Read the model definition and answer for the solid it produces. Units are mm, in the model's axes. Face numbers are marked on the shaded views. A direction names the side the tool comes from. Coordinates: 2 decimals unless noted, no trailing zeros. Write each loop counter-clockwise with the first axis right and the second up, starting at its lowest first coordinate (ties: lowest second). Pieces come first, ordered by that corner, then holes.
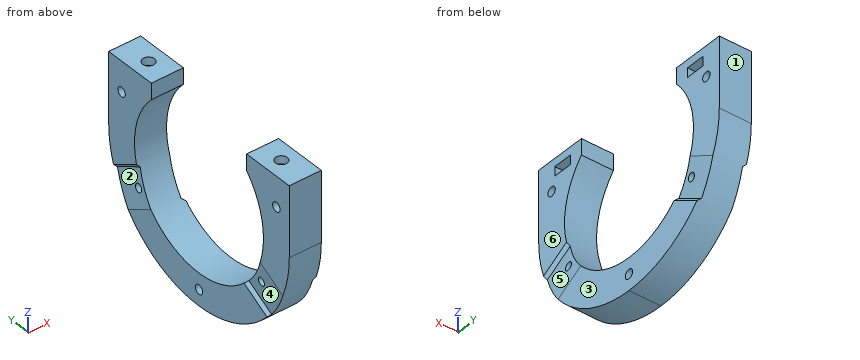
from build123d import *

# Parameters (mm, degrees)
PAD006_DEPTH          = 12
SKETCH077_R           = 1.725
HOLE036_DEPTH         = 12.001
SKETCH067_R           = 2.2
POCKET040_DEPTH       = 12
POCKET041_DEPTH       = 3.5
SKETCH027_R           = 1.5
POCKET042_DEPTH       = 227.579227
POCKET042_DEPTH_BACK  = 228.768023
POCKET043_DEPTH       = 275.16353
POLARPATTERN003_COUNT = 2
POLARPATTERN003_ANGLE = 240


with BuildPart() as part:
    # Sketch021 → Pad006 (new body)
    with BuildSketch(Plane.YZ):
        with BuildLine():
            Line((-42, 26.25), (-22.134532, 26.25))
            Line((-22.134532, 26.25), (-22.134532, 20.25))
            ThreePointArc((-22.134532, 20.25), (0, -30), (22.134532, 20.25))
            Line((22.134532, 26.25), (22.134532, 20.25))
            Line((22.134532, 26.25), (42, 26.25))
            Line((42, 26.25), (42, 7.3e-05))
            ThreePointArc((0, -42), (29.698511, -29.698459), (42, 7.3e-05))
            ThreePointArc((-42, 7.2e-05), (-29.69851, -29.69846), (0, -42))
            Line((-42, 26.25), (-42, 7.2e-05))
        make_face()
    extrude(amount=PAD006_DEPTH)

    # Sketch077 (on DatumPlane) → Hole036 (cut, through all)
    with BuildSketch(Plane.YZ.offset(12)):
        with Locations((0, -36)):
            Circle(SKETCH077_R)
        with Locations((-36, 15)):
            Circle(SKETCH077_R)
        with Locations((36, 15)):
            Circle(SKETCH077_R)
    extrude(amount=-HOLE036_DEPTH, mode=Mode.SUBTRACT)

    # Sketch067 (on DatumPlane) → Pocket040 (cut)
    with BuildSketch(Plane(origin=(6, 0, 26.25), x_dir=(1, 0, 0), z_dir=(0, 0, 1))):
        with Locations((0, 30.875)):
            Circle(SKETCH067_R)
        with Locations((0, -30.875)):
            Circle(SKETCH067_R)
    extrude(amount=-POCKET040_DEPTH, mode=Mode.SUBTRACT)

    # Sketch068 (on DatumPlane) → Pocket041 (cut)
    with BuildSketch(Plane(origin=(6, 0, 23.25), x_dir=(1, 0, 0), z_dir=(0, 0, 1))):
        Polygon((-2.107328, -27.225), (-4.214657, -30.875), (-2.107328, -34.525), (9.892672, -34.525), (9.892672, -27.225), align=None)
        Polygon((-2.107328, 34.525), (-4.214657, 30.875), (-2.107328, 27.225), (9.892672, 27.225), (9.892672, 34.525), align=None)
    extrude(amount=-POCKET041_DEPTH, mode=Mode.SUBTRACT)

    # Sketch027 (on DatumPlane) → Pocket042 (cut, two sides)
    with BuildSketch(Plane(origin=(6, 0, 0), x_dir=(0.087156, 0.498097, 0.86273), z_dir=(0.996195, -0.043578, -0.075479))) as pocket042_sk:
        with Locations((0, -33)):
            Circle(SKETCH027_R)
    pocket042 = extrude(amount=-POCKET042_DEPTH, mode=Mode.SUBTRACT) + extrude(pocket042_sk.sketch, amount=POCKET042_DEPTH_BACK, mode=Mode.SUBTRACT)

    # Sketch066 (on DatumPlane) → Pocket043 (cut, through all)
    with BuildSketch(Plane(origin=(6, 0, 0), x_dir=(1, 0, 0), z_dir=(0, -0.866025, 0.5))):
        Polygon((6, 5.999897), (7, 5.999897), (7, -9.083659), (4.866975, -6.950634), align=None)
        Polygon((-7, 9.083659), (-4.866975, 6.950634), (-6, -5.999897), (-7, -5.999897), align=None)
    pocket043 = extrude(amount=-POCKET043_DEPTH, mode=Mode.SUBTRACT)

    # PolarPattern003: Pocket043, Pocket042 ×2 about axis
    polarpattern003_axis = Axis((0, 0, 0), (1, 0, 0))
    for i in range(1, POLARPATTERN003_COUNT):
        add(pocket043.rotate(polarpattern003_axis, i * POLARPATTERN003_ANGLE / (POLARPATTERN003_COUNT - 1)), mode=Mode.SUBTRACT)
        add(pocket042.rotate(polarpattern003_axis, i * POLARPATTERN003_ANGLE / (POLARPATTERN003_COUNT - 1)), mode=Mode.SUBTRACT)


with BuildPart() as part_1:
    # Body022004 placement: moved
    add(part.part.moved(Location((123, 0, 834))))


solid = part_1.part
Item 1: Determine the mould class of the marked faces 1, 2 and 3 for opening direction Y: +Y half, -Y half, draft (parallel to the pull), parting line (faces both ways), or undercut.
Item 2: For the marked faces 4, 5 and 6, determine the directions among +Z, -Z, +X, -X, +Y, -Y from which every point of the face is accessible in a straight line to the end or side of a thin tool.
Item 3: Given pin 1 (1.5 mm diameter, centred on x = 132.5, y = -12, fed in from -Z); pin 2 (5 mm diameter, centred on x = 129.5, y = 12.5, fed in from -Z); pin 3 (2 mm diameter, centred on y = 36, z = 849, fed in from -X); pin 4 (7 mm diameter, centred on x = 129, y = 30.875, fed in from -Z), each flat-ended and moving along its own axis, determine where each tip first touches the part or whether it passes through.
Item 4: The part is cut by section D-D (x = 129). State how many separate pieces and enclosed holes the cut face has, and give its area (3 significant figures).
Item 5: The part is cut by section B-B (y = 36). Give the vertices of the cut face in (x, z) (3 decimals).
Item 6: Find the intervals of material crossed by probe 1 along Y at (x, z) = (130.5, 855.5) (3 decimals); probe 2 along Y at (x, z) = (124.5, 849) (3 decimals); probe 3 along Y at (x, z) = (133, 843), in increasing order.
Item 7: The part is cut by section A-A (z = 798). Give the vertices of the cut face in (x, y) (3 decimals), and give its area (3 significant figures).
Item 8: The part is cut by section C-C (z = 837.5). Give the vertices of the cut face in (x, y).
Answer:
1. face 1: +Y half
1. face 2: undercut
1. face 3: draft
2. face 4: -X
2. face 5: +X
2. face 6: +Z, -Z, +X, +Y, -Y
3. pin 1: stops at z = 793.53
3. pin 2: stops at z = 793.21
3. pin 3: passes through
3. pin 4: stops at z = 802.15
4. separate pieces: 1
4. enclosed holes: 5
4. area: 2,010 mm2
5. outline: (123, 822.55) - (124.133, 821.241) - (123.461, 812.367) - (134.411, 812.367) - (135, 820.143) - (135, 847.275) - (123, 847.275) - close; (123, 850.725) - (135, 850.725) - (135, 860.25) - (123, 860.25) - close
6. probe 1: y = -42 to -34.525, -27.225 to -22.135, 22.135 to 27.225, 34.525 to 42
6. probe 2: y = -42 to -37.725, -34.275 to -25.981, 25.981 to 34.275, 37.725 to 42
6. probe 3: y = -42 to -28.62, 28.62 to 42
7. outline: (123, -21.633) - (135, -21.633) - (135, -1.725) - (123, -1.725) - close; (123, 1.725) - (135, 1.725) - (135, 21.633) - (123, 21.633) - close
7. area: 478 mm2
8. outline: (123, -42) - (135, -42) - (135, -29.8) - (123, -29.8) - close; (123, 29.8) - (135, 29.8) - (135, 42) - (123, 42) - close
